For this review, take the finished solid that the model builds, in its own axes (mm). A direction names the side the tool comes from. Coordinates: 2 decimals unless noted, no trailing zeros. Write each loop counter-clockwise with the first axis right and the second up, starting at its lowest first coordinate (ties: lowest second). Pieces come first, ordered by that corner, then holes. Notation, with made-up numbers: M 47.5,-6.75 L 74.5,-6.75 A14 cw 74.5,1.25 Z; hole C 53.25,21.25 d10. An arc over 180 degrees is marked long. One line per question, with ' | ' between items.
from build123d import *

# Parameters (mm, degrees)
SKETCH1_R           = 1.5875
BOSS_EXTRUDE1_DEPTH = 1.6


with BuildPart() as part:
    # Sketch1 → Boss-Extrude1 (new, symmetric)
    with BuildSketch(Plane.XY):
        with BuildLine():
            Line((19.545643943, -2.5), (-19.545643943, -2.5))
            Line((-19.545643943, -2.5), (-24.328510099, -3.434981996))
            ThreePointArc((-24.328510099, -3.434981996), (-28.5, 0), (-24.328510099, 3.434981996))
            Line((-24.328510099, 3.434981996), (-19.545643943, 2.5))
            Line((-19.545643943, 2.5), (19.545643943, 2.5))
            Line((19.545643943, 2.5), (24.328510099, 3.434981996))
            ThreePointArc((24.328510099, 3.434981996), (28.5, 0), (24.328510099, -3.434981996))
            Line((24.328510099, -3.434981996), (19.545643943, -2.5))
        make_face()
        with Locations((-25, 0)):
            Circle(SKETCH1_R, mode=Mode.SUBTRACT)
        with Locations((25, 0)):
            Circle(SKETCH1_R, mode=Mode.SUBTRACT)
    extrude(amount=BOSS_EXTRUDE1_DEPTH, both=True)


solid = part.part
1) We need section D-D on x = -19. State the section outline as (y, z) points, then the cut area to 3 significant figures.
Responses:
outline: M -2.5,-1.6 L 2.5,-1.6 L 2.5,1.6 L -2.5,1.6 Z | area: 16.0 mm^2
2) Machinability: for faces 4 (the cylindrical face through (26.514, 0.477, -0.022)), 5 (the flat face through (21.971, -2.974, 0.022)), 6 (the flat face through (-21.971, 2.974, 0.022)), which of the approach directions +Z, -Z, +X, -X, +Y, -Y give a long, thin tool a straight path to every point of the face, cutting with its end or side? Answer none if there is none.
Responses:
face 4: +Z, -Z | face 5: +Z, -Z, -Y | face 6: +Z, -Z, +Y
3) The part is to be moulded in two halves that separate along Y. For faces 1 (the flat face through (0, 0, -1.6)), 2 (the flat face through (-21.9, -2.96, 0.02)), 3 (the cylindrical face through (-23.486, 0.477, -0.022)), say which applies: +Y half, -Y half, draft (parallel to the pull), parting line (faces both ways), or undercut.
Responses:
face 1: draft | face 2: -Y half | face 3: undercut
4) We need section B-B on z = -0.95. State the section outline as (x, y) points (1 decimal).
Responses:
outline: M -24.3,-3.4 L -19.5,-2.5 L 19.5,-2.5 L 24.3,-3.4 A3.5 ccw long 24.3,3.4 L 19.5,2.5 L -19.5,2.5 L -24.3,3.4 A3.5 ccw long Z; hole C -25,0 d3.2; hole C 25,0 d3.2
5) To check wall thickness, follow line 1 along Y through (x, z) = (25, -0.8); line 2 along Y through (x, z) = (6.5, 1.3); line 3 along X through (y, z) = (-0.75, 0.05). State the ranges of each line that lie inside material, in increasing order. Write a range as [from, to].
Responses:
line 1: [-3.5, -1.59], [1.59, 3.5] | line 2: [-2.5, 2.5] | line 3: [-28.42, -26.4], [-23.6, 23.6], [26.4, 28.42]
6) We need section C-C on x = -25. State the section outline as (y, z) points, then the cut area to 3 significant figures.
Responses:
outline: M -3.5,-1.6 L -1.59,-1.6 L -1.59,1.6 L -3.5,1.6 Z; M 1.59,-1.6 L 3.5,-1.6 L 3.5,1.6 L 1.59,1.6 Z | area: 12.2 mm^2
7) Insertion check: pin 1 Ø1.9 at (x, y) = (-25, 0) entering from +Z; pin 2 Ø1 at (x, z) = (7, 0) entering from -Y. Each pin has a flat end and moves straight along its axis. Give the tip position at first contact, or say it passes through.
Responses:
pin 1: through | pin 2: y = -2.5
8) We need section A-A on y = 0. State the section outline as (x, z) points.
Responses:
outline: M -28.5,-1.6 L -26.59,-1.6 L -26.59,1.6 L -28.5,1.6 Z; M -23.41,-1.6 L 23.41,-1.6 L 23.41,1.6 L -23.41,1.6 Z; M 26.59,-1.6 L 28.5,-1.6 L 28.5,1.6 L 26.59,1.6 Z
